Verification items for the finished model (mm, model axes). Face numbers are marked on the shaded views. A direction names the side the tool comes from. Give positions to 0.01 mm unless a question says otherwise; leave off trailing zeros. Order: outer loops, then holes, each group sorted by start corner. A loop starts at its lowest first (then second) coordinate and runs counter-clockwise, first axis right, second up.
(1) Access from +Z, -Z, +X, -X, +Y, -Y to the whole of each face (thin tool, end or side, straight path). Record for the marked faces 1 and 2.
(2) Gauge pin test, flat ends, axial feed: pin 1 (1.5 mm diameter, centred on y = -52, z = -8, fed in from +X); pin 2 (4 mm diameter, centred on x = 3.5, y = -33, fed in from -Z); pin 3 (1 mm diameter, centred on y = 1, z = 9.5, fed in from +X); pin 4 (0.6 mm diameter, centred on y = 2, z = -10, fed in from +X). Record the tip position at first contact, or that the pin passes through.
(3) Sectioned sample at A-A on z = 0. Record the cut outline in (x, y) (3 decimals).
(4) Scan lines: L1, parallel to Y at x = -2.75, z = -8.75 (3 decimals); L2, parallel to X at y = -37, z = -6.25; L3, parallel to Z at x = 8.75, y = -3.5. Record each from-to range of solid material in increasing order.
(5) Sectioned sample at C-C on y = -59. Record the cut outline in (x, z), plus the area to 3 significant figures.
(6) Sectioned sample at B-B on y = -39.5. Record the cut outline in (x, z).
(7) Sectioned sample at D-D on z = 6. Record the cut outline in (x, y) (3 decimals).
```python
from build123d import *

# Parameters (mm, degrees)
F0_R     = 12.7
F1_DEPTH = 53.975
F2_R     = 3.5
F3_DEPTH = 2
F5_DEPTH = 10
F6_W     = 0.5
F6_H     = 2
F7_DEPTH = 3
F8_R     = 0.5
F9_DEPTH = 25.4


with BuildPart() as f1:
    # F0 (on Front) → F1 (new body)
    with BuildSketch(Plane.XZ):
        Circle(F0_R)
    extrude(amount=F1_DEPTH)

    # F2 (on face) → F3 (join)
    with BuildSketch(Plane.XZ.offset(53.975)):
        Circle(F2_R)
    extrude(amount=F3_DEPTH)

    # F4 (on face) → F5 (join)
    with BuildSketch(Plane.XZ.offset(55.975)):
        with BuildLine():
            Line((-0.962927, 1.752932), (-0.962927, -1.752932))
            ThreePointArc((-0.962927, -1.752932), (2, 0), (-0.962927, 1.752932))
        make_face()
    extrude(amount=F5_DEPTH)

    # F6 (on face) → F7 (join)
    with BuildSketch(Plane(origin=(0, 0, 0), x_dir=(-1, 0, 0), z_dir=(0, 1, 0))):
        with Locations((0.004237, 10.055495)):
            Rectangle(F6_W, F6_H)
        with Locations((0.004237, -10.055495)):
            Rectangle(F6_W, F6_H)
    extrude(amount=F7_DEPTH)

    # F8 (on face) → F9 (cut)
    with BuildSketch(Plane(origin=(-0.254237, 0, 0), x_dir=(0, -1, 0), z_dir=(-1, 0, 0))):
        with Locations((-1.627872, 10.00566)):
            Circle(F8_R)
        with Locations((-1.892378, -10.130965)):
            Circle(F8_R)
    extrude(amount=-F9_DEPTH, mode=Mode.SUBTRACT)


solid = f1.part
```
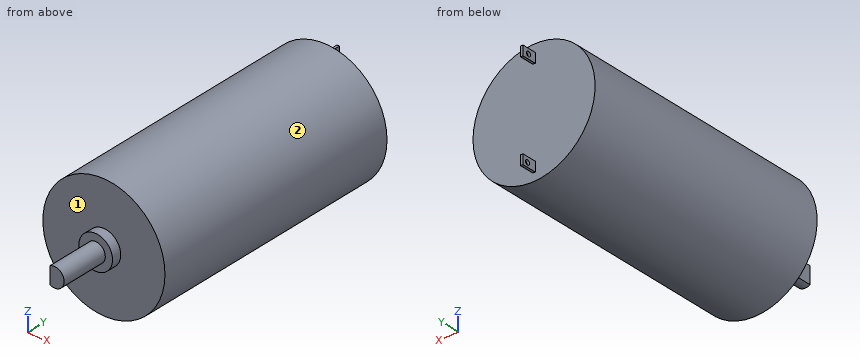
Ans:
1. face 1: -Y
1. face 2: +Y, -Y
2. pin 1: stops at x = 10.43
2. pin 2: stops at z = -12.61
2. pin 3: stops at x = 0.25
2. pin 4: passes through
3. outline: (-12.7, -53.975) - (-3.5, -53.975) - (-3.5, -55.975) - (-0.963, -55.975) - (-0.963, -65.975) - (2, -65.975) - (2, -55.975) - (3.5, -55.975) - (3.5, -53.975) - (12.7, -53.975) - (12.7, 0) - (-12.7, 0) - close
4. L1: y = -53.975 to 0
4. L2: x = -11.06 to 11.06
4. L3: z = -9.2 to 9.2
5. outline: (-0.96, -1.75) arc R2 ccw (long way) to (-0.96, 1.75) - close
5. area: 9.98 mm2
6. outline: circle Ø25.4 at (0, 0)
7. outline: (-11.193, -53.975) - (11.193, -53.975) - (11.193, 0) - (-11.193, 0) - close
